Build history of the part. All positions in model axes, mm. A direction names the side the tool comes from. Coordinates: 2 decimals unless noted, no trailing zeros. Order: outer loops, then holes, each group sorted by start corner. A loop starts at its lowest first (then second) coordinate and runs counter-clockwise, first axis right, second up. Notation, with made-up numbers: (66, 45) - (82, 45) arc R19 cw to (82, 79) - close; hole circle Ø9 at (68, 38.5). An arc over 180 degrees is marked (long way). Answer as CSV lines item,"result". Start each with the question number.
from build123d import *

# Parameters (mm, degrees)
SKETCH1_R           = 1.525
SKETCH1_R_2         = 1.025
SKETCH1_W           = 70
SKETCH1_H           = 8
SKETCH1_W_2         = 3
SKETCH1_H_2         = 5
SKETCH1_W_3         = 10
SKETCH1_H_3         = 20
SKETCH1_W_4         = 15
SKETCH1_H_4         = 14
SKETCH1_W_5         = 12.6
SKETCH1_H_5         = 18.75
BOSS_EXTRUDE1_DEPTH = 3


with BuildPart() as part:
    # Sketch1 → Boss-Extrude1 (new body)
    with BuildSketch(Plane(origin=(0, 0, 0), x_dir=(1, 0, 0), z_dir=(0, 1, 0))):
        Polygon((0, 0), (130, 0), (130, -92.5), (130, -97.5), (130, -120), (0, -120), (0, -97.5), (0, -92.5), align=None)
        with Locations(Location((28.2, -115, 0), (0, 0, 270))):
            Circle(SKETCH1_R, mode=Mode.SUBTRACT)
        with Locations(Location((101.8, -115, 0), (0, 0, 270))):
            Circle(SKETCH1_R, mode=Mode.SUBTRACT)
        with Locations(Location((121.5, -90, 0), (0, 0, 270))):
            Circle(SKETCH1_R, mode=Mode.SUBTRACT)
        with Locations(Location((8.5, -90, 0), (0, 0, 270))):
            Circle(SKETCH1_R, mode=Mode.SUBTRACT)
        with Locations(Location((78.06, -90, 0), (0, 0, 270))):
            Circle(SKETCH1_R, mode=Mode.SUBTRACT)
        with Locations(Location((51.94, -90, 0), (0, 0, 270))):
            Circle(SKETCH1_R, mode=Mode.SUBTRACT)
        with Locations(Location((124, -107, 0), (0, 0, 270))):
            Circle(SKETCH1_R, mode=Mode.SUBTRACT)
        with Locations(Location((6, -107, 0), (0, 0, 270))):
            Circle(SKETCH1_R, mode=Mode.SUBTRACT)
        with Locations(Location((30, -75, 0), (0, 0, 270))):
            Circle(SKETCH1_R, mode=Mode.SUBTRACT)
        with Locations(Location((30, -16.71, 0), (0, 0, 270))):
            Circle(SKETCH1_R, mode=Mode.SUBTRACT)
        with Locations(Location((56.4, -75, 0), (0, 0, 270))):
            Circle(SKETCH1_R, mode=Mode.SUBTRACT)
        with Locations(Location((86, -70, 0), (0, 0, 270))):
            Circle(SKETCH1_R_2, mode=Mode.SUBTRACT)
        with Locations(Location((86, -54.77, 0), (0, 0, 270))):
            Circle(SKETCH1_R_2, mode=Mode.SUBTRACT)
        with Locations(Location((79, -16, 0), (0, 0, 270))):
            Circle(SKETCH1_R, mode=Mode.SUBTRACT)
        with Locations(Location((109.24, -32.38, 0), (0, 0, 270))):
            Circle(SKETCH1_R, mode=Mode.SUBTRACT)
        with Locations(Location((18, -115, 0), (0, 0, 270))):
            Circle(SKETCH1_R, mode=Mode.SUBTRACT)
        with Locations(Location((112, -115, 0), (0, 0, 270))):
            Circle(SKETCH1_R, mode=Mode.SUBTRACT)
        with Locations(Location((5, -5, 0), (0, 0, 270))):
            Circle(SKETCH1_R, mode=Mode.SUBTRACT)
        with Locations(Location((125, -5, 0), (0, 0, 270))):
            Circle(SKETCH1_R, mode=Mode.SUBTRACT)
        with Locations((65, -108)):
            Rectangle(SKETCH1_W, SKETCH1_H, mode=Mode.SUBTRACT)
        with Locations((3.5, -95)):
            Rectangle(SKETCH1_W_2, SKETCH1_H_2, mode=Mode.SUBTRACT)
        with Locations((102.5, -62.5)):
            Rectangle(SKETCH1_W_3, SKETCH1_H_3, mode=Mode.SUBTRACT)
        with Locations((112, -44.38)):
            Rectangle(SKETCH1_W_4, SKETCH1_H_4, mode=Mode.SUBTRACT)
        with Locations((11.3, -39.375)):
            Rectangle(SKETCH1_W_5, SKETCH1_H_5, mode=Mode.SUBTRACT)
    extrude(amount=BOSS_EXTRUDE1_DEPTH)


solid = part.part
(1) Pull direction Z, two halves, no side cores. Call faces 3 (the flat face through (130, 1, 61)), 4 (the flat face through (66, 1, 120)), 5 (the flat face through (119.5, 1, 44)): +Z half, -Z half, draft (parallel to the pull), parting line (faces both ways), or undercut.
(2) Band-saw the part on C-C on x = 96. List the corners of the cut face in (y, z).
(3) Band-saw the part on B-B on z = 94. List the corners of the cut face in (x, y).
(4) Which spindle directions (+Z, -Z, +X, -X, +Y, -Y) get a long thin tool onto all of the face, cutting with end or side? Do faces 1 (the flat face through (66, 3, 59)), 2 (the flat face through (112, 1, 51.38)). Say none if no direction does.
(5) Band-saw the part on A-A on x = 56.4. List the corners of the cut face in (y, z) (3 decimals).
(6) Band-saw the part on D-D on y = 2.25. State how many separate pieces and enclosed holes the cut face has, plus the area to 3 significant figures.
(7) Probe L1, parallel to X at y = 1.95, z = 54.77 (3 decimals); L2, parallel to Z at x = 86, y = 2 (3 decimals); L3, parallel to X at y = 0.85, z = 75 (3 decimals). List the from-to ranges inside material, lowest first. Write a range as [from, to].
Filled in:
1,face 3,"draft"
1,face 4,"+Z half"
1,face 5,"undercut"
2,outline,"(0, 0) - (3, 0) - (3, 104) - (0, 104) - close; (0, 112) - (3, 112) - (3, 120) - (0, 120) - close"
3,outline,"(0, 0) - (2, 0) - (2, 3) - (0, 3) - close; (5, 0) - (130, 0) - (130, 3) - (5, 3) - close"
4,face 1,"+Z, -Z, +X, -X, +Y"
4,face 2,"+Y, -Y"
5,outline,"(0, 0) - (3, 0) - (3, 73.475) - (0, 73.475) - close; (0, 76.525) - (3, 76.525) - (3, 104) - (0, 104) - close; (0, 112) - (3, 112) - (3, 120) - (0, 120) - close"
6,separate pieces,"1"
6,enclosed holes,"24"
6,area,"14,200 mm^2"
7,L1,"x = [0, 84.975], [87.025, 97.5], [107.5, 130]"
7,L2,"z = [0, 53.745], [55.795, 68.975], [71.025, 104], [112, 120]"
7,L3,"x = [0, 28.475], [31.525, 54.875], [57.925, 130]"
